```python
from build123d import *

# Parameters (mm, degrees)
F2_R     = 10
F3_R     = 10.7
F4_DEPTH = 8.7
F5_R     = 0.6
F6_SIZE  = 0.5


with BuildPart() as f1:
    # F0 (on Front) → F1 (revolve)
    with BuildSketch(Plane.XZ):
        Polygon((-8.7, 0), (0, 0), (0, 32.525253), (-9, 32.525253), (-9, 47.45), (-35, 47.45), (-35, 20.825), (-8.7, 20.825), align=None)
    revolve(axis=Axis((-4.35, 0, 0), (-1, 0, 0)))

    # F2
    f2_edges = [f1.edges().sort_by_distance(p)[0] for p in [
        (-35, 0, -47.45),
    ]]
    fillet(f2_edges, radius=F2_R)

    # F3 (on face) → F4 (cut, through all)
    with BuildSketch(Plane(origin=(-8.7, 0, 0), x_dir=(0, -1, 0), z_dir=(-1, 0, 0))):
        Circle(F3_R)
    extrude(amount=-F4_DEPTH, mode=Mode.SUBTRACT)

    # F5
    f5_edges = [f1.edges().sort_by_distance(p)[0] for p in [
        (-8.7, 0, -20.825),
        (-9, 0, -32.525253),
    ]]
    fillet(f5_edges, radius=F5_R)

    # F6
    f6_edges = [f1.edges().sort_by_distance(p)[0] for p in [
        (-9, 0, -47.45),
        (0, 0, -32.525253),
        (0, 10.7, 0),
        (-8.7, 10.7, 0),
        (-35, 0, -20.825),
    ]]
    chamfer(f6_edges, length=F6_SIZE)


solid = f1.part
```
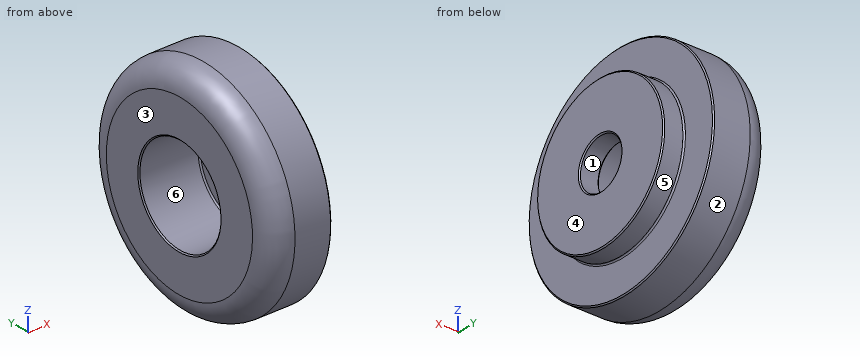
Geometry check sheet. Reference: the model listing, model coordinates, mm. Face numbers are marked on the shaded views. A direction names the side the tool comes from. Coordinates: 2 decimals unless noted, no trailing zeros. Write each loop counter-clockwise with the first axis right and the second up, starting at its lowest first coordinate (ties: lowest second). Pieces come first, ordered by that corner, then holes. Notation, with made-up numbers: M 42.25,-10.75 L 60.25,-10.75 A32 cw 60.25,16.25 Z; hole C 88,64.5 d10. An arc over 180 degrees is marked long. One line per item, written item: value. Start each with the question number.
(1) Depth check by flat-ended pin: pin 1 (1 mm diameter, centred on x = -12, y = -27, fed in from +Z); pin 2 (24.5 mm diameter, centred on y = 0, z = 0, fed in from -X); pin 3 (5 mm diameter, centred on x = -26.5, z = -10.5, fed in from -Y); pin 4 (12 mm diameter, centred on y = -24.5, z = 32.5, fed in from -X). Enter the tip coordinate at first touch or a pass-through.
(2) Scan lines: line 1 along Z through (x, y) = (-2, 0.5); line 2 along Y through (x, z) = (-25, 0) (3 decimals); line 3 along Y through (x, z) = (-12.5, -2). Record each from-to range of solid material in increasing order. Write a range as [from, to].
(3) Sectioned sample at D-D, the plane x = -6. Enter the section's corners in (y, z).
(4) Release check for a two-part mould opening along Z. For the marked faces 1, 2 and 3 record: released by +Z, released by -Z, zero draft, split by the parting line, or undercut.
(5) Tool access check on the marked faces 4, 5 and 6. Record the directions out of +Z, -Z, +X, -X, +Y, -Y that give a thin tool (end or side, any length) a straight path to the whole face; none if there is none.
(6) Sectioned sample at C-C, the plane x = -22. Enter the section's corners in (y, z) (3 decimals).
Filled sheet:
1. pin 1: z = 39.36
1. pin 2: x = -8.7
1. pin 3: y = -46.72
1. pin 4: x = -35
2. line 1: [-32.52, -10.69], [10.69, 32.52]
2. line 2: [-47.45, -20.825], [20.825, 47.45]
2. line 3: [-47.41, -20.73], [20.73, 47.41]
3. outline: C 0,0 d65.05; hole C 0,0 d21.4
4. face 1: undercut
4. face 2: split by the parting line
4. face 3: zero draft
5. face 4: +Z, -Z, +X, +Y, -Y
5. face 5: +X
5. face 6: -X
6. outline: C 0,0 d94.9; hole C 0,0 d41.65
